Can you work these out from the model? Positions are in its coordinate system, mm. Face numbers are marked on the shaded views. Give positions to 0.01 mm unless a question says otherwise; leave off trailing zeros. Order: outer loops, then holes, each group sorted by start corner. A loop starts at its lowest first (then second) coordinate and runs counter-clockwise, first axis right, second up. Notation, with made-up numbers: M 87,74.25 L 92,74.25 A27 cw 92,102.25 Z; hole C 49.5,44.5 d5. An arc over 180 degrees is marked long. Use a Markdown table: item, result. Add a question column.
Autodesk Inventor part; units mm, degrees
ref_plane "YZ Plane" through (0, 0, 0) normal (1, 0, 0) x (0, 1, 0)
ref_plane "XZ Plane" through (0, 0, 0) normal (0, 1, 0) x (-1, 0, 0)
ref_plane "XY Plane" through (0, 0, 0) normal (0, 0, 1) x (1, 0, 0)
sketch "Sketch1" plane through (0, 0, 0) normal (0, 0, 1) x (1, 0, 0)
  circle A0 centre (48.2493, -30.8623) radius 2.1844
  circle A1 centre (57.5164, -22.1784) radius 2.1844
  circle A2 centre (5.4131, 33.4246) radius 2.1844
  circle A3 centre (-3.854, 24.7407) radius 2.1844
  circle A4 centre (22.4893, 5.9147) radius 2.1844
  circle A5 centre (-57.1544, -5.4775) radius 2.1844 construction
  circle A6 centre (-57.1544, -18.1775) radius 2.1844 construction
  arc A7 (-60.5073, -0.0848) -> (-63.5044, -5.4775) centre (-57.1544, -5.4775) ccw
  arc A8 (-63.5044, -18.1775) -> (-57.9131, -24.482) centre (-57.1544, -18.1775) ccw
  circle A9 centre (-57.1544, -5.4775) radius 2.1844
  circle A10 centre (-57.1544, -18.1775) radius 2.1844
  arc A11 (10.0467, 37.7665) -> (2.0602, 38.8172) centre (5.4131, 33.4246) ccw
  arc A12 (61.8584, -26.812) -> (62.15, -17.8364) centre (57.5164, -22.1784) ccw
  arc A13 (47.4906, -37.1668) -> (52.5912, -35.4958) centre (48.2493, -30.8623) ccw
  line L0 (10.0467, 37.7665) -> (62.15, -17.8364)
  line L1 (61.8584, -26.812) -> (52.5912, -35.4958)
  line L2 (47.4906, -37.1668) -> (-57.9131, -24.482)
  line L3 (-63.5044, -18.1775) -> (-63.5044, -5.4775)
  line L4 (-60.5073, -0.0848) -> (2.0602, 38.8172)
  circle A14 centre (-25.4044, -11.8275) radius 2.1844
  dimension "d0" = 12.7
  dimension "d1" = 12.7
  dimension "d2" = 12.7
  dimension "d3" = 12.7
  dimension "d4" = 12.7
  dimension "d7" = 4.3688
  dimension "d8" = 31.75
  dimension "d9" = 6.35
extrude "Extrusion1" add sketch "Sketch1" along normal blind 1.5875
properties part number "2.1-Gearbox"
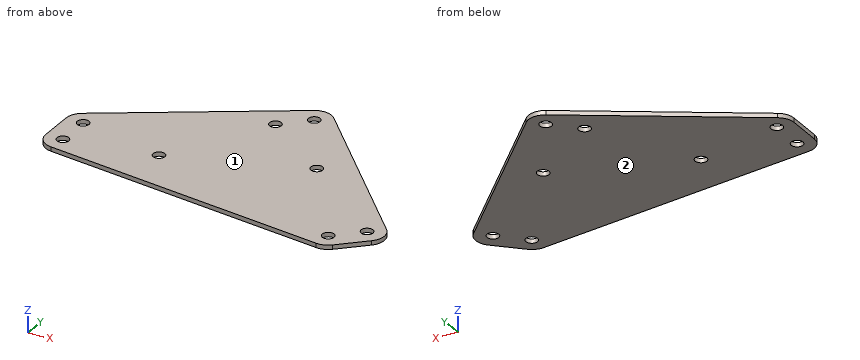
1. If we section it at B-B, the plane x = 40: List the corners of the cut face in (y, z) for me.
2. If we section it at A-A, the plane z = 0.8: State how many separate pieces and enclosed holes the cut face has, then the cut area to 3 significant figures.
3. I need wall thicknesses on L1, parallel to X at y = -13, z = 0.9; L2, parallel to Y at x = 15, z = 1.3; L3, parallel to X at y = -22, z = 1.3 (1 decimal). Which ranges of each line are inside material? Lowest first, please. Write a range as [from, to].
4. We'd pull the mould along Z, two halves only. Please class the marked faces 1 and 2: +Z half, -Z half, draft (parallel to the pull), parting line (faces both ways), or undercut.
5. If we section it at C-C, the plane y = 14.5: List the corners of the cut face in (x, z) for me, then the cut area to 3 significant figures.
Geometry results:
| question | item | result |
|---|---|---|
| 1 | outline | M -36.27,0 L 5.8,0 L 5.8,1.59 L -36.27,1.59 Z |
| 2 | separate pieces | 1 |
| 2 | enclosed holes | 8 |
| 2 | area | 5,790 mm^2 |
| 3 | L1 | x = [-63.5, -27.25], [-23.56, 57.62] |
| 3 | L2 | y = [-33.26, 32.48] |
| 3 | L3 | x = [-62.2, 55.3], [59.7, 63.9] |
| 4 | face 1 | +Z half |
| 4 | face 2 | -Z half |
| 5 | outline | M -37.05,0 L 31.85,0 L 31.85,1.59 L -37.05,1.59 Z |
| 5 | area | 109 mm^2 |
